Could you check a few things on this drawing? It's one solid part, dimensions in mm from its lowest x, y, z. Give positions to 0.01 mm unless a question says otherwise; leave off trailing zeros. Write each loop counter-clockwise with the first axis right and the second up, starting at its lowest first coordinate (ties: lowest second). Pieces come first, ordered by that corner, then holes. Notation, with made-up numbers: (-36, 33) -> (13, 33) arc R23 cw to (13, 50) -> close; hole circle Ø7 at (-31.75, 6). An arc over 180 degrees is marked (long way). Answer as CSV lines item,"result". Start each with the question number.
1. I'm going to push flat-ended pins straight in: P1, Ø5, axis at y = 2.5, z = 158, coming from the +X side; P2, Ø4, axis at x = 22.5, z = 123.5, coming from the -Y side. Where does each tip first touch, or does it pass through?
2. I need wall thicknesses on line 1 (Z direction, x = 12.75, y = 10); line 2 (X direction, y = 18.25, z = 17); line 3 (Z direction, x = 14.75, y = 1.75). Which ranges of each line are inside material? Lowest first, please. Write a range as [from, to].
3. If we section it at B-B on x = 12.7: Write out the boundary of the cut face in (y, z), plus the area to 3 significant figures.
4. If we section it at D-D on z = 27.5: Write out the boundary of the cut face in (x, y).
5. If we section it at C-C on y = 17.5: Write out the boundary of the cut face in (x, z).
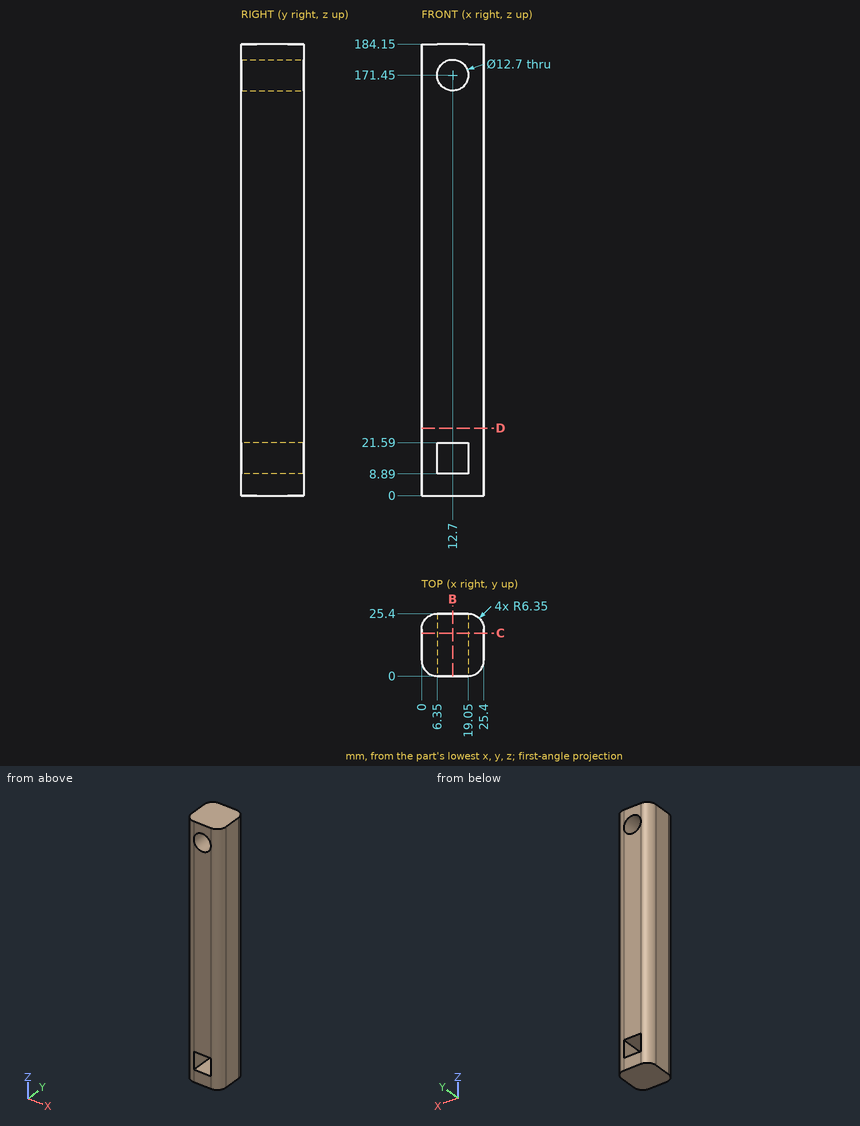
Computed values:
1,P1,"stops at x = 25.25"
1,P2,"stops at y = 0.17"
2,line 1,"z = [0, 8.89], [21.59, 165.1], [177.8, 184.15]"
2,line 2,"x = [0, 6.35], [19.05, 25.4]"
2,line 3,"z = [0, 8.89], [21.59, 165.44], [177.46, 184.15]"
3,outline,"(0, 0) -> (25.4, 0) -> (25.4, 8.89) -> (0, 8.89) -> close; (0, 21.59) -> (25.4, 21.59) -> (25.4, 165.1) -> (0, 165.1) -> close; (0, 177.8) -> (25.4, 177.8) -> (25.4, 184.15) -> (0, 184.15) -> close"
3,area,"4,030 mm2"
4,outline,"(0, 6.35) arc R6.35 ccw to (6.35, 0) -> (19.05, 0) arc R6.35 ccw to (25.4, 6.35) -> (25.4, 19.05) arc R6.35 ccw to (19.05, 25.4) -> (6.35, 25.4) arc R6.35 ccw to (0, 19.05) -> close"
5,outline,"(0, 0) -> (25.4, 0) -> (25.4, 184.15) -> (0, 184.15) -> close; hole (6.35, 8.89) -> (19.05, 8.89) -> (19.05, 21.59) -> (6.35, 21.59) -> close; hole circle Ø12.7 at (12.7, 171.45)"
